Check sheet for the modelled part. Datum: model origin and axes. Units: mm. Face numbers are marked on the shaded views. A direction names the side the tool comes from. Round coordinates to 2 decimals unless told otherwise and drop trailing zeros. Order: outer loops, then holes, each group sorted by start corner. A loop starts at its lowest first (then second) coordinate and runs counter-clockwise, first axis right, second up.
(1) Mould release check, pull along Y, two halves, no side actions. Record for the marked faces 1, 2 and 3: released by +Y, released by -Y, zero draft, split by the parting line, or undercut.
(2) Sectioned sample at A-A, the plane y = 7.5. Count the separate pieces of the cut face and the enclosed holes in it, and give its area (3 significant figures).
(3) Sectioned sample at B-B, the plane z = 24.5. Enter the section's corners in (x, y).
(4) Tool access check on the marked faces 4 and 5. Record the directions out of +Z, -Z, +X, -X, +Y, -Y that give a thin tool (end or side, any length) a straight path to the whole face; none if there is none.
(5) Thickness scan on probe 1 along X at (y, z) = (6.75, -2.5); probe 2 along Z at (x, y) = (-13, 6.25); probe 3 along X at (y, z) = (13, 4). Record the ranges inside material, lowest first.
(6) Depth check by flat-ended pin: pin 1 (3 mm diameter, centred on y = 10.5, z = -8, fed in from -X); pin 2 (1 mm diameter, centred on y = 7.5, z = -1.5, fed in from +X); pin 3 (10 mm diameter, centred on x = -22.5, y = 12.5, fed in from +Z); pin 4 (4 mm diameter, centred on y = 8.5, z = -17.5, fed in from -X). Enter the tip coordinate at first touch or a pass-through.
```python
from build123d import *
from OCP.BRepFilletAPI import BRepFilletAPI_MakeChamfer

# Parameters (mm, degrees)
BOSS_EXTRUDE1_DEPTH     = 15
SKETCH2_R               = 3.05
CUT_EXTRUDE1_DEPTH      = 15
BOSS_EXTRUDE2_DEPTH     = 5
CHAMFER4_SIZE           = 3
CHAMFER6_SIZE           = 15
CHAMFER6_SIZE_2         = 2
CUT_EXTRUDE2_DEPTH      = 29
CUT_EXTRUDE2_DEPTH_BACK = 25
SKETCH4_R               = 1.5
SKETCH5_R               = 2.5
CUT_EXTRUDE3_DEPTH      = 14.024984395
CUT_EXTRUDE4_START      = -14.024984395
SKETCH6_R               = 2.5
CUT_EXTRUDE4_DEPTH      = 14.024984395


with BuildPart() as part:
    # Sketch1 → Boss-Extrude1 (new body)
    with BuildSketch(Plane(origin=(0, 0, 0), x_dir=(1, 0, 0), z_dir=(0, 1, 0))):
        with BuildLine():
            ThreePointArc((-14.719179189, 14.619614321), (-15.719179189, -9.839501126), (-16.719179189, 14.619614321))
            Line((-16.719179189, 14.619614321), (-16.719179189, 22.410498874))
            ThreePointArc((-16.719179189, 22.410498874), (-35.465683849, 5.738494325), (-23.219179189, -16.156945753))
            Line((-23.219179189, -16.156945753), (-23.219179189, -31.156945753))
            Line((-23.219179189, -31.156945753), (-8.219179189, -31.156945753))
            Line((-8.219179189, -31.156945753), (-8.219179189, -16.156945753))
            ThreePointArc((-8.219179189, -16.156945753), (4.02732547, 5.738494325), (-14.719179189, 22.410498874))
            Line((-14.719179189, 22.410498874), (-14.719179189, 14.619614321))
        make_face()
    extrude(amount=BOSS_EXTRUDE1_DEPTH)

    # Sketch2 → Cut-Extrude1 (cut)
    with BuildSketch(Plane.XY.offset(31.156945753)):
        with Locations((-15.719179189, 7.5)):
            Circle(SKETCH2_R)
    extrude(amount=-CUT_EXTRUDE1_DEPTH, mode=Mode.SUBTRACT)

    # Sketch3 → Boss-Extrude2 (add)
    with BuildSketch(Plane(origin=(0, 15, 0), x_dir=(1, 0, 0), z_dir=(0, 1, 0))):
        with BuildLine():
            Line((-16.719179189, 14.619614321), (-16.719179189, 17.377128421))
            ThreePointArc((-16.719179189, 17.377128421), (-25.966129955, -8.543952276), (-0.719179189, 2.410498874))
            ThreePointArc((-0.719179189, 2.410498874), (-4.764728039, 12.65744964), (-14.719179189, 17.377128421))
            Line((-14.719179189, 17.377128421), (-14.719179189, 14.619614321))
            ThreePointArc((-14.719179189, 14.619614321), (-6.710502816, 10.711477732), (-3.469179189, 2.410498874))
            ThreePointArc((-3.469179189, 2.410498874), (-24.020158047, -6.598177499), (-16.719179189, 14.619614321))
        make_face()
    extrude(amount=BOSS_EXTRUDE2_DEPTH)

    # Chamfer4
    chamfer4_edges = [part.edges().sort_by_distance(p)[0] for p in [
        (-25.966129955, 15, 8.543952276),
        (-35.465683849, 0, -5.738494325),
        (4.02732547, 0, -5.738494325),
    ]]
    chamfer(chamfer4_edges, length=CHAMFER4_SIZE)

    # Chamfer6
    chamfer6_edges_1 = [part.edges().sort_by_distance(p)[0] for p in [
        (-23.219179189, 7.5, 31.156945753),
    ]]
    chamfer6_side_1 = [part.faces().sort_by_distance(p)[0] for p in [
        (-23.219179189, 7.5, 31.116945753),
    ]]
    chamfer6_edges_2 = [part.edges().sort_by_distance(p)[0] for p in [
        (-8.219179189, 7.5, 31.156945753),
    ]]
    chamfer6_side_2 = [part.faces().sort_by_distance(p)[0] for p in [
        (-8.259179189, 7.5, 31.156945753),
    ]]
    chamfer6_edges_3 = [part.edges().sort_by_distance(p)[0] for p in [
        (-15.719179189, 15, 31.156945753),
    ]]
    chamfer6_side_3 = [part.faces().sort_by_distance(p)[0] for p in [
        (-15.719179189, 14.96, 31.156945753),
    ]]
    chamfer6 = BRepFilletAPI_MakeChamfer(part.part.solid().wrapped)
    for e in chamfer6_edges_1:
        chamfer6.Add(CHAMFER6_SIZE - 0.0001, CHAMFER6_SIZE_2 - 0.0001, e.wrapped, chamfer6_side_1[0].wrapped)
    for e in chamfer6_edges_2:
        chamfer6.Add(CHAMFER6_SIZE_2 - 0.0001, CHAMFER6_SIZE - 0.0001, e.wrapped, chamfer6_side_2[0].wrapped)
    for e in chamfer6_edges_3:
        chamfer6.Add(CHAMFER6_SIZE_2 - 0.0001, CHAMFER6_SIZE - 0.0001, e.wrapped, chamfer6_side_3[0].wrapped)
    add(Compound.cast(chamfer6.Shape()), mode=Mode.REPLACE)  # a hair under: the kernel refuses the full size

    # Sketch4 → Cut-Extrude2 (cut, two sides: drawn at the far end of the back side and taken through both)
    with BuildSketch(Plane.ZY.offset(14.719179189).offset(-CUT_EXTRUDE2_DEPTH_BACK)):
        with Locations(Location((-17.410498874, 7.5, 0), (0, 0, 180))):
            Circle(SKETCH4_R)
    extrude(amount=CUT_EXTRUDE2_DEPTH + CUT_EXTRUDE2_DEPTH_BACK, mode=Mode.SUBTRACT)

    # Sketch5 → Cut-Extrude3 (cut)
    with BuildSketch(Plane(origin=(4.305805205, 0, 0), x_dir=(0, 0, -1), z_dir=(1, 0, 0))):
        with Locations((17.410498874, 7.5)):
            Circle(SKETCH5_R)
    extrude(amount=-CUT_EXTRUDE3_DEPTH, mode=Mode.SUBTRACT)

    # Sketch6 → Cut-Extrude4 (cut)
    with BuildSketch(Plane.ZY.offset(35.744163584).offset(CUT_EXTRUDE4_START)):
        with Locations(Location((-17.410498874, 7.5, 0), (0, 0, 180))):
            Circle(SKETCH6_R)
    extrude(amount=CUT_EXTRUDE4_DEPTH, mode=Mode.SUBTRACT)


solid = part.part
```
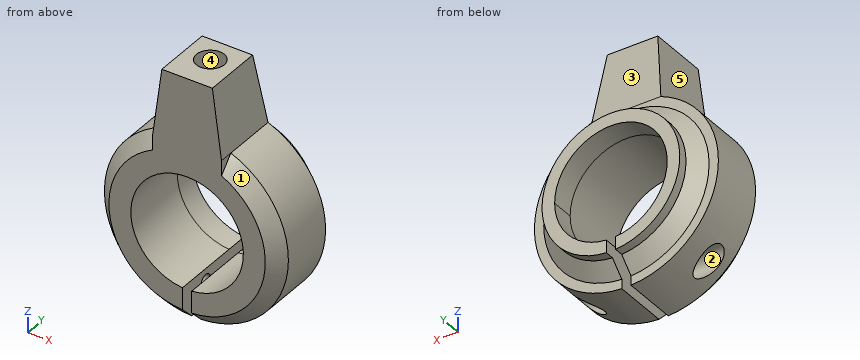
Derived:
1. face 1: released by -Y
1. face 2: undercut
1. face 3: released by +Y
2. separate pieces: 3
2. enclosed holes: 0
2. area: 761 mm2
3. outline: (-22.11, 0) - (-9.33, 0) - (-9.33, 13.89) - (-22.11, 13.89) - close; hole circle Ø6.1 at (-15.72, 7.5)
4. face 4: +Z
4. face 5: +Z, -X, +Y, -Y
5. probe 1: x = -35.74 to -27.97, -3.47 to 4.31
5. probe 2: z = -22.25 to -18.24, -16.58 to -14.35, 9.53 to 16.16
5. probe 3: x = -34.69 to -26.16, -5.28 to 3.25
6. pin 1: stops at x = -35.32
6. pin 2: stops at x = 4.3
6. pin 3: stops at z = 31.16
6. pin 4: stops at x = -30.73
